Verification items for this drawing (mm, ordinates from the low corner). Round coordinates to 2 decimals unless told otherwise and drop trailing zeros. Loops run counter-clockwise (first coordinate to the right, second up) from the corner with the lowest first, then second, coordinate; pieces in that order, holes last. Notation, with made-up numbers: (32.5, -38) -> (63.5, -38) arc R17 cw to (63.5, -13) -> close; hole circle Ø3 at (62, -2.75). An arc over 180 degrees is marked (long way). One line per question, with ' | ' between items.
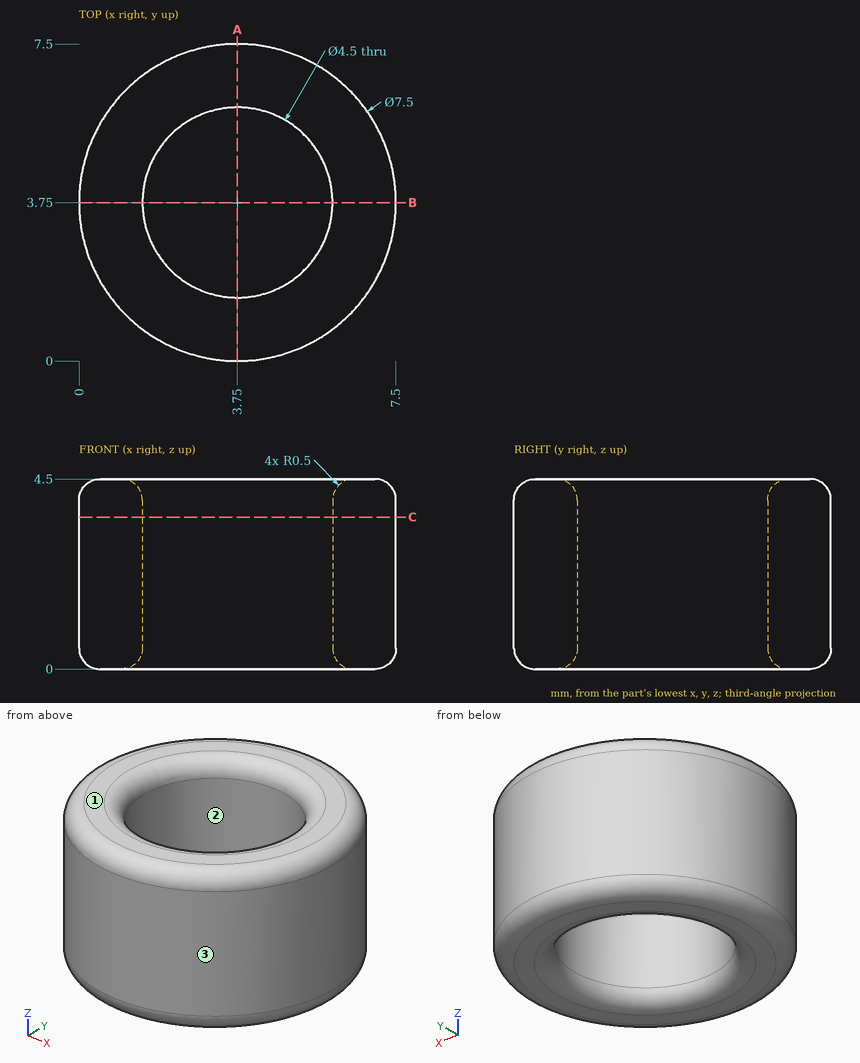
(1) Mould release check, pull along Y, two halves, no side actions. Record for the marked faces 1, 2 and 3: +Y half, -Y half, draft (parallel to the pull), parting line (faces both ways), or undercut.
Answer:
face 1: draft | face 2: undercut | face 3: parting line
(2) Scan lines: probe 1 along Y at (x, z) = (3.75, 2); probe 2 along Y at (x, z) = (1.75, 1.3); probe 3 along X at (y, z) = (2, 3.55). Record each from-to range of solid material in increasing order.
Answer:
probe 1: y = 0 to 1.5, 6 to 7.5 | probe 2: y = 0.58 to 2.72, 4.78 to 6.92 | probe 3: x = 0.43 to 2.34, 5.16 to 7.07
(3) Sectioned sample at C-C, the plane z = 3.6. Record the cut outline in (x, y), and give its area (3 significant figures).
Answer:
outline: circle Ø7.5 at (3.75, 3.75); hole circle Ø4.5 at (3.75, 3.75) | area: 28.3 mm2
(4) Sectioned sample at A-A, the plane x = 3.75. Record the cut outline in (y, z), and give its area (3 significant figures).
Answer:
outline: (0, 0.5) arc R0.5 ccw to (0.5, 0) -> (1, 0) arc R0.5 ccw to (1.5, 0.5) -> (1.5, 4) arc R0.5 ccw to (1, 4.5) -> (0.5, 4.5) arc R0.5 ccw to (0, 4) -> close; (6, 0.5) arc R0.5 ccw to (6.5, 0) -> (7, 0) arc R0.5 ccw to (7.5, 0.5) -> (7.5, 4) arc R0.5 ccw to (7, 4.5) -> (6.5, 4.5) arc R0.5 ccw to (6, 4) -> close | area: 13.1 mm2
(5) Go/stop test with flat-tipped pins: pin 1 (2 mm diameter, centred on x = 5, z = 2, fed in from +Y); pin 2 (1 mm diameter, centred on y = 6.5, z = 4, fed in from -X); pin 3 (2 mm diameter, centred on x = 6.5, z = 1.5, fed in from +Y). Record where each tip stops, or that it passes through.
Answer:
pin 1: stops at y = 7.49 | pin 2: stops at x = 0.75 | pin 3: stops at y = 7.07
